Source: CAD feature listing. Evaluate the final solid. Frame: model axes, mm. Face numbers are marked on the shaded views. Give positions to 0.01 mm unless a question says otherwise; leave off trailing zeros. Order: outer loops, then holes, each group sorted by start corner. A loop starts at its lowest first (then second) coordinate and runs counter-clockwise, first axis right, second up. Notation, with made-up numbers: (-39, 85.5) -> (-28, 85.5) arc R12 cw to (-28, 90.5) -> close; hole circle Ø7 at (86, -26). An arc over 180 degrees is marked (long way). Use CSV: the item, a comma, the result in double quotes.
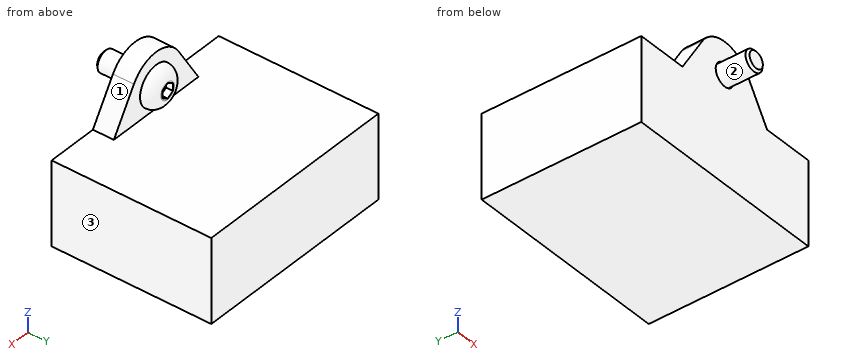
```python
from build123d import *

# Parameters (mm, degrees)
SKETCH_1_W          = 39.5
SKETCH_1_H          = 16
EXTRUDE_1_DEPTH     = 30.5
EXTRUDE_2_DEPTH     = 4
SKETCH_3_W          = 2.15
SKETCH_3_H          = 4
CUT_EXTRUDE_1_DEPTH = 1.3


with BuildPart() as part:
    # Sketch 1 → Extrude 1 (new body)
    with BuildSketch(Plane(origin=(0, 0, 0), x_dir=(1, 0, 0), z_dir=(0, 1, 0))):
        with Locations((0, 8)):
            Rectangle(SKETCH_1_W, SKETCH_1_H)
    extrude(amount=EXTRUDE_1_DEPTH)

    # Sketch 2 → Extrude 2 (add)
    with BuildSketch(Plane(origin=(0, 0, 0), x_dir=(1, 0, 0), z_dir=(0, 1, 0))):
        with BuildLine():
            Line((-10, 0), (-5.257226723, -7.586573775))
            ThreePointArc((-5.257226723, -7.586573775), (0, -10.5), (5.257226723, -7.586573775))
            Line((5.257226723, -7.586573775), (10, 0))
            Line((10, 0), (-10, 0))
        make_face()
    extrude(amount=EXTRUDE_2_DEPTH)

    # Sketch 3 → Cut-Revolve 1 (revolve, cut)
    with BuildSketch(Plane.XY.offset(4.3), mode=Mode.PRIVATE) as cut_revolve_1_sk:
        with Locations((1.075, 2)):
            Rectangle(SKETCH_3_W, SKETCH_3_H)
    revolve(cut_revolve_1_sk.sketch.rotate(Axis((0, 0, 4.3), (0, 1, 0)), 270), axis=Axis((0, 0, 4.3), (0, 1, 0)), mode=Mode.SUBTRACT)

    # Sketch 4 → Revolve 1 (revolve)
    with BuildSketch(Plane.XY.offset(4.3), mode=Mode.PRIVATE) as revolve_1_sk:
        with BuildLine():
            Line((0, 6.2), (1.6, 6.2))
            ThreePointArc((1.6, 6.2), (3.155634919, 5.555634919), (3.8, 4))
            Line((3.8, 4), (2, 4))
            Line((2, 4), (2, -5.5705))
            Line((2, -5.5705), (1.5705, -6))
            Line((1.5705, -6), (0, -6))
            Line((0, -6), (0, 6.2))
        make_face()
    revolve(revolve_1_sk.sketch.rotate(Axis((0, -6, 4.3), (0, 1, 0)), 270), axis=Axis((0, -6, 4.3), (0, 1, 0)))

    # Sketch 5 → Cut-Extrude 1 (cut)
    with BuildSketch(Plane(origin=(0, 6.2, 0), x_dir=(1, 0, 0), z_dir=(0, 1, 0))):
        Polygon((-1.25, -3.578312164), (-1.25, -5.021687836), (0, -5.743375673), (1.25, -5.021687836), (1.25, -3.578312164), (0, -2.856624327), align=None)
    extrude(amount=-CUT_EXTRUDE_1_DEPTH, mode=Mode.SUBTRACT)


solid = part.part
```
1. Mould query, pull axis Z, two halves, no side actions, for the marked faces 1, 2 and 3. Classes: released by +Z, released by -Z, zero draft, split by the parting line, or undercut.
Answer below:
face 1,"released by +Z"
face 2,"undercut"
face 3,"zero draft"
2. Section query C-C on x = -16. Return loops of the section in (y, z).
Answer below:
outline,"(0, -16) -> (30.5, -16) -> (30.5, 0) -> (0, 0) -> close"
3. Section query A-A on z = -6.75. Return loops of the section in (x, y).
Answer below:
outline,"(-19.75, 0) -> (19.75, 0) -> (19.75, 30.5) -> (-19.75, 30.5) -> close"
4. Ray query, line 1 along Z through (x, y) = (-3.5, 25.5); line 2 along X through (y, z) = (1, 4.25); line 3 along Y through (x, z) = (1.5, -9.5). Return the intervals inside material, ascending.
Answer below:
line 1,"z = -16 to 0"
line 2,"x = -7.34 to -2.15, -2 to 2, 2.15 to 7.34"
line 3,"y = 0 to 30.5"
5. Pin query (flat end, axial travel): P1, Ø1.5, axis at x = -15, y = 4.5, coming from the +Z side; P2, Ø8, axis at y = 1.5, z = 7, coming from the -X side; P3, Ø2.5, axis at x = 0, z = 4.5, coming from the +Y side. Return the tip coordinate at first contact, or that it passes through.
Answer below:
P1,"stops at z = 0"
P2,"stops at x = -8.12"
P3,"stops at y = 6.2"
6. Section query B-B on y = -3. Return loops of the section in (x, z), plus the area to 3 significant figures.
Answer below:
outline,"circle Ø4 at (0, 4.3)"
area,"12.6 mm²"
